```python
from build123d import *

# Parameters (mm, degrees)
F1_DEPTH = 8
F3_DEPTH = 6
F4_R     = 0.5


with BuildPart() as f1:
    # F0 (on Top) → F1 (new body)
    with BuildSketch(Plane.XY):
        Polygon((8.082904, 0), (4.041452, 7), (-4.041452, 7), (-8.082904, 0), (-4.041452, -7), (4.041452, -7), align=None)
    extrude(amount=F1_DEPTH)

    # F2 (on face) → F3 (cut)
    with BuildSketch(Plane.XY.offset(8)):
        with BuildLine():
            Line((3.2, -3.2), (3.2, 3.2))
            Line((3.2, 3.2), (-3.2, 3.2))
            Line((-3.2, 3.2), (-3.2, -3.2))
            Line((-3.2, -3.2), (-1, -3.2))
            Line((-1, -3.2), (-1, -1.7))
            ThreePointArc((-1, -1.7), (0, -0.7), (1, -1.7))
            Line((1, -1.7), (1, -3.2))
            Line((1, -3.2), (3.2, -3.2))
        make_face()
    extrude(amount=-F3_DEPTH, mode=Mode.SUBTRACT)

    # F4
    f4_edges = [f1.edges().sort_by_distance(p)[0] for p in [
        (-6.062178, -3.5, 0),
        (0, -7, 0),
        (6.062178, -3.5, 0),
        (6.062178, 3.5, 0),
        (0, 7, 0),
        (-6.062178, 3.5, 0),
        (0, -7, 8),
        (6.062178, -3.5, 8),
        (6.062178, 3.5, 8),
        (0, 7, 8),
        (-6.062178, 3.5, 8),
        (-6.062178, -3.5, 8),
    ]]
    fillet(f4_edges, radius=F4_R)


solid = f1.part
```
Verification items for the finished model (mm, model axes). A direction names the side the tool comes from. Give positions to 0.01 mm unless a question says otherwise; leave off trailing zeros. Order: outer loops, then holes, each group sorted by start corner. A loop starts at its lowest first (then second) coordinate and runs counter-clockwise, first axis right, second up. Notation, with made-up numbers: (-1, 80) -> (33, 80) arc R20 ccw to (33, 93) -> close; hole circle Ø1 at (65, 44). An arc over 180 degrees is marked (long way). Use a Markdown table: item, result.
1) Mould release check, pull along X, two halves, no side actions. Record for faces 3 (the flat face through (3.2, 0, 5)), 4 (the flat face through (-6.09, -3.45, 3.95)), 5 (the flat face through (6.034, -3.549, 3.951)): pulls with the +X half, pulls with the -X half, needs draft (parallel to the pull), parting line crosses it, or undercut.
Results:
| item | result |
|---|---|
| face 3 | undercut |
| face 4 | pulls with the -X half |
| face 5 | pulls with the +X half |
2) Material ranges on probe 1 along Y at (x, z) = (1.5, 4); probe 2 along X at (y, z) = (-1.5, 3.25); probe 3 along Z at (x, y) = (1.5, -0.5), recorded low to high.
Results:
| item | result |
|---|---|
| probe 1 | -7 to -3.2, 3.2 to 7 |
| probe 2 | -7.22 to -3.2, -0.98 to 0.98, 3.2 to 7.22 |
| probe 3 | 0 to 2 |
3) Depth check by flat-ended pin: pin 1 Ø1.8 at (y, z) = (1, 6) entering from +X; pin 2 Ø0.8 at (y, z) = (-2.5, 5.5) entering from +X; pin 3 Ø0.5 at (y, z) = (-2.5, 6) entering from -X. Enter the tip coordinate at first touch or a pass-through.
Results:
| item | result |
|---|---|
| pin 1 | x = 8.03 |
| pin 2 | x = 6.87 |
| pin 3 | x = -6.78 |
4) Section check B-B, the plane x = 0. Record the boundary of the cut face in (y, z).
Results:
| item | result |
|---|---|
| outline | (-7, 0.5) arc R0.5 ccw to (-6.5, 0) -> (6.5, 0) arc R0.5 ccw to (7, 0.5) -> (7, 7.5) arc R0.5 ccw to (6.5, 8) -> (3.2, 8) -> (3.2, 2) -> (-0.7, 2) -> (-0.7, 8) -> (-6.5, 8) arc R0.5 ccw to (-7, 7.5) -> close |
5) Section check D-D, the plane x = 2.75. Record the boundary of the cut face in (y, z), then the cut area to 3 significant figures.
Results:
| item | result |
|---|---|
| outline | (-7, 0.5) arc R0.5 ccw to (-6.5, 0) -> (6.5, 0) arc R0.5 ccw to (7, 0.5) -> (7, 7.5) arc R0.5 ccw to (6.5, 8) -> (3.2, 8) -> (3.2, 2) -> (-3.2, 2) -> (-3.2, 8) -> (-6.5, 8) arc R0.5 ccw to (-7, 7.5) -> close |
| area | 73.4 mm² |
6) Section check A-A, the plane z = 4.5. Record the boundary of the cut face in (x, y).
Results:
| item | result |
|---|---|
| outline | (-8.08, 0) -> (-4.04, -7) -> (4.04, -7) -> (8.08, 0) -> (4.04, 7) -> (-4.04, 7) -> close; hole (-3.2, -3.2) -> (-1, -3.2) -> (-1, -1.7) arc R1 cw to (1, -1.7) -> (1, -3.2) -> (3.2, -3.2) -> (3.2, 3.2) -> (-3.2, 3.2) -> close |
7) Section check C-C, the plane z = 1.25. Record the boundary of the cut face in (x, y), then the cut area to 3 significant figures.
Results:
| item | result |
|---|---|
| outline | (-8.08, 0) -> (-4.04, -7) -> (4.04, -7) -> (8.08, 0) -> (4.04, 7) -> (-4.04, 7) -> close |
| area | 170 mm² |
8) Tool access check on faces 1 (the cylindrical face through (0, -0.7, 5)), 2 (the flat face through (0, -1, 8)). Record the directions out of +Z, -Z, +X, -X, +Y, -Y that give a thin tool (end or side, any length) a straight path to the whole face; none if there is none.
Results:
| item | result |
|---|---|
| face 1 | +Z |
| face 2 | +Z, +X, -X, +Y, -Y |
